The model under review builds one solid part; all positions refer to its coordinate system, in mm. Face numbers are marked on the shaded views. A direction names the side the tool comes from. Round coordinates to 2 decimals unless told otherwise and drop trailing zeros. Loops run counter-clockwise (first coordinate to the right, second up) from the corner with the lowest first, then second, coordinate; pieces in that order, holes last. Notation, with made-up numbers: M 79,62 L 114,62 A20 ccw 114,69 Z; hole C -9,74 d5. An arc over 180 degrees is marked long. Answer as a JSON object with one key per item and string values. Group by question number.
Item 1: Consider section A-A (y = 14.5). Give the boundary of the cut face in (x, z), and give its area (3 significant figures).
Item 2: Consider section C-C (y = 64.5). Give the boundary of the cut face in (x, z), and give its area (3 significant figures).
Item 3: To check wall thickness, follow line 1 (Z direction, x = -90, y = 61.75); line 2 (X direction, y = 3, z = 7.25); line 3 (X direction, y = 39, z = 9.25). State the ranges of each line that lie inside material, in increasing order.
Item 4: Consider section D-D (z = 4.75). Give the boundary of the cut face in (x, y), and give its area (3 significant figures).
Item 5: Tool access review of the marked faces 1 and 2: name each direction out of +Z, -Z, +X, -X, +Y, -Y from which nothing blocks a thin tool from reaching the whole face with its end or side.
Item 6: Insertion check: P1, Ø0.8, axis at x = -0.5, y = 49, coming from the -Z side; P2, Ø1.8, axis at x = -113, z = 9, coming from the -Y side; P3, Ø3, axis at y = 30, z = 17, coming from the -X side; P4, Ø4, axis at x = -12, z = 9.5, coming from the -Y side. Each pin has a flat end and moves straight along its axis. Give the tip position at first contact, or say it passes through.
Item 7: Consider section B-B (x = -90). Give the boundary of the cut face in (y, z).
```python
from build123d import *

# Parameters (mm, degrees)
BOSS_EXTRUDE1_DEPTH = 20
SKETCH2_W           = 5.1
SKETCH2_H           = 40
CUT_EXTRUDE1_DEPTH  = 20
FILLET1_R           = 7
CUT_EXTRUDE3_REACH  = 155.379
SKETCH5_R           = 3.7
SKETCH6_W           = 87.272363661
SKETCH6_H           = 5
CUT_EXTRUDE4_DEPTH  = 3
FILLET2_R           = 3
SKETCH7_W           = 3
SKETCH7_H           = 5
CUT_EXTRUDE5_DEPTH  = 70
FILLET3_R           = 2


with BuildPart() as part:
    # Sketch1 → Boss-Extrude1 (new body)
    with BuildSketch(Plane.XY):
        Polygon((0, 0), (0, 70), (-135, 70), (-135, 55), (-25, 55), (-25, 0), align=None)
    extrude(amount=BOSS_EXTRUDE1_DEPTH)

    # Sketch2 → Cut-Extrude1 (cut)
    with BuildSketch(Plane.XY.offset(20)):
        with Locations((-12.5, 20)):
            Rectangle(SKETCH2_W, SKETCH2_H)
    extrude(amount=-CUT_EXTRUDE1_DEPTH, mode=Mode.SUBTRACT)

    # Fillet1
    fillet1_edges = [part.edges().sort_by_distance(p)[0] for p in [
        (-80, 55, 20),
        (-80, 55, 0),
    ]]
    fillet(fillet1_edges, radius=FILLET1_R)

    # Cut-Extrude3: up to this face of the body (flat: up to its plane)
    cut_extrude3_end = Plane(part.part.faces().sort_by_distance((-80, 55, 10))[0])
    # Sketch5 → Cut-Extrude3 (cut, up to the picked face)
    with BuildSketch(Plane(origin=(0, 70, 0), x_dir=(1, 0, 0), z_dir=(0, 1, 0)), mode=Mode.PRIVATE) as cut_extrude3_sk1:
        with Locations(Location((-90, -10, 0), (0, 0, 180))):
            Circle(SKETCH5_R)
    cut_extrude3_tool1 = split(extrude(cut_extrude3_sk1.sketch, amount=-CUT_EXTRUDE3_REACH, mode=Mode.PRIVATE), bisect_by=cut_extrude3_end, keep=Keep.BOTH, mode=Mode.PRIVATE)
    add(cut_extrude3_tool1.solids().sort_by(Axis((-90, 70, 10), (0, -1, 0)))[0], mode=Mode.SUBTRACT)

    # Sketch6 → Cut-Extrude4 (cut)
    with BuildSketch(Plane(origin=(0, 70, 0), x_dir=(1, 0, 0), z_dir=(0, 1, 0))):
        with Locations((-43.63618183, -10)):
            Rectangle(SKETCH6_W, SKETCH6_H)
    extrude(amount=-CUT_EXTRUDE4_DEPTH, mode=Mode.SUBTRACT)

    # Fillet2
    # the kernel refuses this fillet: 3 mm, written as the material it adds along each edge
    with BuildSketch(Plane(origin=(0, 67, 12.5), x_dir=(0, 0, -1), z_dir=(-1, 0, 0))) as fillet2_piece_1_section:
        with BuildLine():
            CenterArc((FILLET2_R, -FILLET2_R), FILLET2_R, 90, 90)
            Line((0, -FILLET2_R), (0, 0))
            Line((0, 0), (FILLET2_R, 0))
        make_face()
    fillet2_piece_1 = extrude(amount=94.772363661, mode=Mode.PRIVATE)
    fillet2_piece_1 = fillet2_piece_1 - Plane(origin=(-90, 67.680644159, 10), x_dir=(-1, 0, 0), z_dir=(0, 1, 0)) * Cylinder(3.7, 202, mode=Mode.PRIVATE)
    add(fillet2_piece_1)
    with BuildSketch(Plane(origin=(-94.772363661, 67, 7.5), x_dir=(0, 1, 0), z_dir=(1, 0, 0))) as fillet2_piece_2_section:
        with BuildLine():
            CenterArc((FILLET2_R, FILLET2_R), FILLET2_R, 180, 90)
            Line((0, FILLET2_R), (0, 0))
            Line((0, 0), (FILLET2_R, 0))
        make_face()
    fillet2_piece_2 = extrude(amount=94.772363661, mode=Mode.PRIVATE)
    fillet2_piece_2 = fillet2_piece_2 - Plane(origin=(-90, 67.756833616, 10), x_dir=(-1, 0, 0), z_dir=(0, 1, 0)) * Cylinder(3.7, 202, mode=Mode.PRIVATE)
    add(fillet2_piece_2)

    # Sketch7 → Cut-Extrude5 (cut)
    with BuildSketch(Plane(origin=(0, 70, 0), x_dir=(1, 0, 0), z_dir=(0, 1, 0))):
        with Locations((-1.5, -10)):
            Rectangle(SKETCH7_W, SKETCH7_H)
    extrude(amount=-CUT_EXTRUDE5_DEPTH, mode=Mode.SUBTRACT)

    # Fillet3
    # the kernel refuses this fillet: 2 mm, written as the material it adds along each edge
    with BuildSketch(Plane(origin=(-3, 70, 12.5), x_dir=(0, 0, -1), z_dir=(0, -1, 0))) as fillet3_piece_1_section:
        with BuildLine():
            CenterArc((FILLET3_R, FILLET3_R), FILLET3_R, 180, 90)
            Line((0, FILLET3_R), (0, 0))
            Line((0, 0), (FILLET3_R, 0))
        make_face()
    fillet3_piece_1 = extrude(amount=70, mode=Mode.PRIVATE)
    fillet3_piece_1 = fillet3_piece_1 - Plane(origin=(-2.544196541, 70, 9.5), x_dir=(0, 0, -1), z_dir=(1, 0, 0)) * Cylinder(3, 148, mode=Mode.PRIVATE)
    add(fillet3_piece_1)
    with BuildSketch(Plane(origin=(-3, 70, 7.5), x_dir=(0, 0, 1), z_dir=(0, -1, 0))) as fillet3_piece_2_section:
        with BuildLine():
            CenterArc((FILLET3_R, -FILLET3_R), FILLET3_R, 90, 90)
            Line((0, -FILLET3_R), (0, 0))
            Line((0, 0), (FILLET3_R, 0))
        make_face()
    fillet3_piece_2 = extrude(amount=70, mode=Mode.PRIVATE)
    fillet3_piece_2 = fillet3_piece_2 - Plane(origin=(-2.544196926, 70, 10.5), x_dir=(0, 1, 0), z_dir=(-1, 0, 0)) * Cylinder(3, 148, mode=Mode.PRIVATE)
    add(fillet3_piece_2)


solid = part.part
```
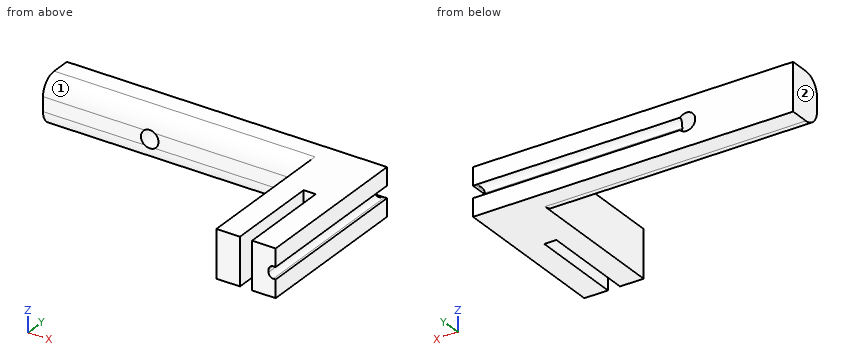
Geometry results:
{
 "1": {"outline": "M -25,0 L -15.05,0 L -15.05,20 L -25,20 Z; M -9.95,0 L 0,0 L 0,7.5 L -1,7.5 A2 cw -3,9.5 L -3,10.5 A2 cw -1,12.5 L 0,12.5 L 0,20 L -9.95,20 Z", "area": "385 mm^2"},
 "2": {"outline": "M -135,0 L 0,0 L 0,7.5 L -1,7.5 A2 cw -3,9.5 L -3,10.5 A2 cw -1,12.5 L 0,12.5 L 0,20 L -135,20 Z; hole C -90,10 d7.4", "area": "2,640 mm^2"},
 "3": {"line 1": "z = 0 to 6.3, 13.7 to 20", "line 2": "x = -25 to -15.05, -9.95 to 0", "line 3": "x = -25 to -15.05, -9.95 to -2.98"},
 "4": {"outline": "M -135,55.37 L -25,55.37 L -25,0 L -15.05,0 L -15.05,40 L -9.95,40 L -9.95,0 L 0,0 L 0,70 L -135,70 Z", "area": "3,160 mm^2"},
 "5": {"face 1": "+Z, -X, -Y", "face 2": "+Z, -Z, -X, +Y, -Y"},
 "6": {"P1": "stops at z = 0", "P2": "stops at y = 55", "P3": "stops at x = -25", "P4": "stops at y = 40"},
 "7": {"outline": "M 55.04,6.3 A7 ccw 62,0 L 70,0 L 70,6.3 Z; M 55.04,13.7 L 70,13.7 L 70,20 L 62,20 A7 ccw Z"}
}
